Job drawing, mm, ordinate dimensions from the low corner. One solid piece. A direction names the side the tool comes from. Round coordinates to 2 decimals unless told otherwise and drop trailing zeros. Order: outer loops, then holes, each group sorted by start corner. A loop starts at its lowest first (then second) coordinate and runs counter-clockwise, first axis right, second up. Notation, with made-up numbers: (38, 38) -> (88, 38) arc R14 cw to (88, 48) -> close; hole circle Ø7 at (84.5, 35). An arc over 180 degrees is marked (long way). Return JSON: item names as keys, results as strings. Group by question number.
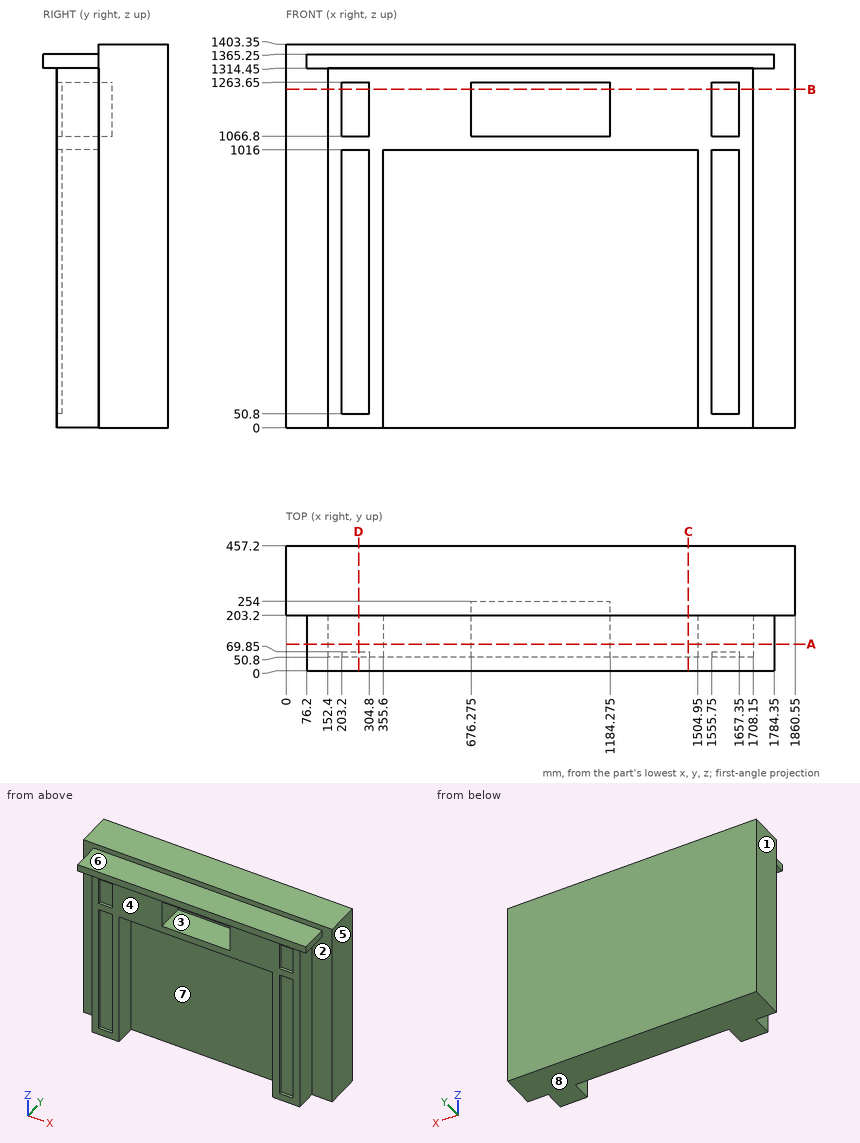
(1) Tool access for the marked faces 4, 5, 6, 7 and 8: list every direction of +Z, -Z, +X, -X, +Y, -Y with a clear straight run to the whole face (end or side of a thin tool).
(2) Pin check, flat tips, straight feed: P1, Ø21, axis at y = 59.5, z = 1138, coming from the +X side; P2, Ø5.5, axis at x = 1614.5, y = 63, coming from the +Z side; P3, Ø5, axis at x = 1143, y = 126.5, coming from the -Z side. Stop position of each tip, or through.
(3) Probe L1, parallel to X at y = 125, z = 589; L2, parallel to Z at x = 854.5, y = 90.5; L3, parallel to Z at x = 641, y = 156. List the from-to ranges inside material, lowest first. Write a range as [from, to].
(4) Saw through at C-C, the plane x = 1471. List the corners of the cut face in (y, z), and give its area (3 significant figures).
(5) Saw through at B-B, the plane z = 1237.5. List the corners of the cut face in (x, y) (3 decimals).
(6) Saw through at A-A, the plane y = 98. List the corners of the cut face in (x, z) (3 decimals).
(7) Saw through at D-D, the plane x = 265. List the corners of the cut face in (y, z).
(8) Mould opens along X. For the marked faces 1, 2 and 3 say: pulls with the +X half, pulls with the -X half, needs draft (parallel to the pull), parting line crosses it, or undercut.
Results are:
{
 "1": {"face 4": "-Z, +X, -X, -Y", "face 5": "+Z, -Z, +X, +Y, -Y", "face 6": "+Z, +X, -X, -Y", "face 7": "-Z, -Y", "face 8": "-Z, +X, -X, +Y, -Y"},
 "2": {"P1": "stops at x = 1708.15", "P2": "stops at z = 1365.25", "P3": "stops at z = 1016"},
 "3": {"L1": "x = [152.4, 355.6], [1504.95, 1708.15]", "L2": "z = [1016, 1066.8], [1263.65, 1365.25]", "L3": "z = [1016, 1365.25]"},
 "4": {"outline": "(0, 1314.45) -> (50.8, 1314.45) -> (50.8, 1016) -> (203.2, 1016) -> (203.2, 0) -> (457.2, 0) -> (457.2, 1403.35) -> (203.2, 1403.35) -> (203.2, 1365.25) -> (0, 1365.25) -> close", "area": "412,000 mm^2"},
 "5": {"outline": "(0, 203.2) -> (152.4, 203.2) -> (152.4, 50.8) -> (203.2, 50.8) -> (203.2, 69.85) -> (304.8, 69.85) -> (304.8, 50.8) -> (676.275, 50.8) -> (676.275, 254) -> (1184.275, 254) -> (1184.275, 50.8) -> (1555.75, 50.8) -> (1555.75, 69.85) -> (1657.35, 69.85) -> (1657.35, 50.8) -> (1708.15, 50.8) -> (1708.15, 203.2) -> (1860.55, 203.2) -> (1860.55, 457.2) -> (0, 457.2) -> close"},
 "6": {"outline": "(76.2, 1314.45) -> (152.4, 1314.45) -> (152.4, 0) -> (355.6, 0) -> (355.6, 1016) -> (1504.95, 1016) -> (1504.95, 0) -> (1708.15, 0) -> (1708.15, 1314.45) -> (1784.35, 1314.45) -> (1784.35, 1365.25) -> (76.2, 1365.25) -> close; hole (676.275, 1066.8) -> (1184.275, 1066.8) -> (1184.275, 1263.65) -> (676.275, 1263.65) -> close"},
 "7": {"outline": "(0, 1314.45) -> (50.8, 1314.45) -> (50.8, 1263.65) -> (69.85, 1263.65) -> (69.85, 1066.8) -> (50.8, 1066.8) -> (50.8, 1016) -> (69.85, 1016) -> (69.85, 50.8) -> (50.8, 50.8) -> (50.8, 0) -> (457.2, 0) -> (457.2, 1403.35) -> (203.2, 1403.35) -> (203.2, 1365.25) -> (0, 1365.25) -> close"},
 "8": {"face 1": "pulls with the -X half", "face 2": "needs draft", "face 3": "undercut"}
}
